The listing builds one solid part. Answer for the finished solid, in the listing's coordinates (mm). A direction names the side the tool comes from. Coordinates: 2 decimals unless noted, no trailing zeros. Write each loop counter-clockwise with the first axis right and the second up, starting at its lowest first coordinate (ties: lowest second). Pieces come first, ordered by that corner, then holes.
from build123d import *

# Parameters (mm, degrees)
BOSS_EXTRUDE1_DEPTH    = 10
SKETCH2_R              = 3
CUT_EXTRUDE1_DEPTH     = 6
SKETCH3_R              = 2.5
BOSS_EXTRUDE2_DEPTH    = 5
SPLIT1_SURFACE_1_BACK  = 134.079
SPLIT1_SURFACE_1_DEPTH = 268.158
SKETCH5_W              = 9.5
SKETCH5_H              = 10
BOSS_EXTRUDE3_DEPTH    = 10
SKETCH6_R              = 2.5
BOSS_EXTRUDE4_DEPTH    = 5
SKETCH7_R              = 3
CUT_EXTRUDE2_DEPTH     = 5
SPLIT3_SURFACE_2_BACK  = 96.932
SPLIT3_SURFACE_2_DEPTH = 193.864


with BuildPart() as part:
    # Sketch1 → Boss-Extrude1 (new body)
    with BuildSketch(Plane(origin=(0, 0, 0), x_dir=(1, 0, 0), z_dir=(0, 1, 0))):
        with BuildLine():
            Line((-57, 0), (-57, -10))
            Line((-57, -10), (-47.5, -10))
            Line((-47.5, -10), (-47.5, 0))
            ThreePointArc((-47.5, 0), (0, 47.5), (47.5, 0))
            Line((47.5, 0), (47.5, -10))
            Line((47.5, -10), (57, -10))
            Line((57, -10), (57, 0))
            ThreePointArc((57, 0), (0, 57), (-57, 0))
        make_face()
    extrude(amount=BOSS_EXTRUDE1_DEPTH)

    # Sketch2 → Cut-Extrude1 (cut)
    with BuildSketch(Plane.XZ):
        with Locations(Location((-52.5, 5, 0), (0, 0, 270))):
            Circle(SKETCH2_R)
    cut_extrude1 = extrude(amount=-CUT_EXTRUDE1_DEPTH, mode=Mode.SUBTRACT)

    # Sketch3 → Boss-Extrude2 (add)
    with BuildSketch(Plane(origin=(0, 10, 0), x_dir=(1, 0, 0), z_dir=(0, 1, 0))):
        with Locations(Location((-52.5, -5, 0), (0, 0, 90))):
            Circle(SKETCH3_R)
    boss_extrude2 = extrude(amount=BOSS_EXTRUDE2_DEPTH)

    # Mirror1: Cut-Extrude1, Boss-Extrude2 across plane
    add(cut_extrude1.mirror(Plane.ZY), mode=Mode.SUBTRACT)
    add(boss_extrude2.mirror(Plane.ZY))

    # Split1: cut with a surface, the side it looks to stays
    # Split1 surface: a surface, the sketch's curves swept straight by 268.158 mm
    with BuildLine(Plane(origin=(0, 10, 0), x_dir=(1, 0, 0), z_dir=(0, 1, 0)).offset(-SPLIT1_SURFACE_1_BACK), mode=Mode.PRIVATE) as split1_surface_1_path:
        Line((0, 47.5), (0, 57))
    split1_surface_1 = Shell.extrude(split1_surface_1_path.wire(), (0 * SPLIT1_SURFACE_1_DEPTH, 1 * SPLIT1_SURFACE_1_DEPTH, 0 * SPLIT1_SURFACE_1_DEPTH))
    split(bisect_by=split1_surface_1, keep=Keep.TOP)

    # Sketch5 → Boss-Extrude3 (add)
    with BuildSketch(Plane(origin=(0, 0, 0), x_dir=(0, 0, -1), z_dir=(1, 0, 0))):
        with Locations((52.25, 5)):
            Rectangle(SKETCH5_W, SKETCH5_H)
    extrude(amount=BOSS_EXTRUDE3_DEPTH)

    # Sketch6 → Boss-Extrude4 (add)
    with BuildSketch(Plane(origin=(0, 10, 0), x_dir=(1, 0, 0), z_dir=(0, 1, 0))):
        with Locations(Location((5, 52.5, 0), (0, 0, 90))):
            Circle(SKETCH6_R)
    extrude(amount=BOSS_EXTRUDE4_DEPTH)

    # Sketch7 → Cut-Extrude2 (cut)
    with BuildSketch(Plane.XZ):
        with Locations(Location((5, -52.5, 0), (0, 0, 270))):
            Circle(SKETCH7_R)
    extrude(amount=-CUT_EXTRUDE2_DEPTH, mode=Mode.SUBTRACT)

    # Split3: cut with a surface, the side it looks to stays
    # Split3 surface: a surface, the sketch's curves swept straight by 193.864 mm
    with BuildLine(Plane(origin=(0, 10, 0), x_dir=(1, 0, 0), z_dir=(0, 1, 0)).offset(-SPLIT3_SURFACE_2_BACK), mode=Mode.PRIVATE) as split3_surface_2_path:
        Line((-49.32, -10), (-49.32, 0))
        ThreePointArc((-49.32, 0), (-34.874506448, 34.874506448), (0, 49.32))
        Line((0, 49.32), (10, 49.32))
    split3_surface_2 = Shell.extrude(split3_surface_2_path.wire(), (0 * SPLIT3_SURFACE_2_DEPTH, 1 * SPLIT3_SURFACE_2_DEPTH, 0 * SPLIT3_SURFACE_2_DEPTH))
    split(bisect_by=split3_surface_2, keep=Keep.TOP)


solid = part.part
Q1. The part is cut by section B-B, the plane y = 4. Write down the section's boundary in (x, z).
Answers below:
outline: (-57, 0) arc R57 ccw to (0, -57) - (10, -57) - (10, -49.32) - (0, -49.32) arc R49.32 cw to (-49.32, 0) - (-49.32, 10) - (-57, 10) - close; hole circle Ø6 at (-52.5, 5); hole circle Ø6 at (5, -52.5)
Q2. The part is cut by section C-C, the plane x = 5. Write down the section's boundary in (y, z).
Answers below:
outline: (0, -57) - (10, -57) - (10, -55) - (15, -55) - (15, -50) - (10, -50) - (10, -49.32) - (0, -49.32) - (0, -49.5) - (5, -49.5) - (5, -55.5) - (0, -55.5) - close
Q3. Given pin 1 (2 mm diameter, centred on x = -46, z = -19.5, fed in from +Y); pin 2 (5 mm diameter, centred on x = 5, z = -52.5, fed in from -Y); pin 3 (5 mm diameter, centred on y = 3, z = 3, fed in from +X), each flat-ended and moving along its own axis, determine where each tip first touches the part or whether it passes through.
Answers below:
pin 1: stops at y = 10
pin 2: stops at y = 5
pin 3: stops at x = -49.32
Q4. Which of the six approach directions +Z, -Z, +X, -X, +Y, -Y give full straight-line access (tool end or side, diameter ignored) to faces 4 (the face through (5, 5, -49.32)), 5 (the face through (-53.251, 12.465, 2.615)), 6 (the face through (5, 5, -52))?
Answers below:
face 4: +Z, +X, +Y, -Y
face 5: +Y
face 6: -Y
Q5. The part is cut by section A-A, the plane z = 5. Write down the section's boundary in (x, y).
Answers below:
outline: (-57, 0) - (-55.5, 0) - (-55.5, 6) - (-49.5, 6) - (-49.5, 0) - (-49.32, 0) - (-49.32, 10) - (-50, 10) - (-50, 15) - (-55, 15) - (-55, 10) - (-57, 10) - close
Q6. Determine the mould class of faces 1 (the face through (-52, 6, 5)), 2 (the face through (5, 15, -52)), 3 (the face through (5, 5, -57)) for opening direction Z: released by +Z, released by -Z, zero draft, split by the parting line, or undercut.
Answers below:
face 1: undercut
face 2: zero draft
face 3: released by -Z
Q7. The part is cut by section D-D, the plane y = 7.5. Write down the section's boundary in (x, z), then the cut area to 3 significant figures.
Answers below:
outline: (-57, 0) arc R57 ccw to (0, -57) - (10, -57) - (10, -49.32) - (0, -49.32) arc R49.32 cw to (-49.32, 0) - (-49.32, 10) - (-57, 10) - close
area: 795 mm2
Q8. Find the intervals of material crossed by probe 1 along X at (y, z) = (4.85, 5); probe 2 along Y at (x, z) = (-46, -25.5); probe 3 along X at (y, z) = (4.05, -52.5), in increasing order.
Answers below:
probe 1: x = -57 to -55.5, -49.5 to -49.32
probe 2: y = 0 to 10
probe 3: x = -22.2 to 2, 8 to 10
